For this review, use the dimensioned drawing (mm, ordinates from the lowest corner) and the shaded views. Coordinates: 2 decimals unless noted, no trailing zeros. Loops run counter-clockwise (first coordinate to the right, second up) from the corner with the lowest first, then second, coordinate; pieces in that order, holes last. Notation, with made-up numbers: M 65.5,-7 L 114.5,-7 A28 ccw 114.5,23 Z; hole C 35,-4.5 d10. An arc over 180 degrees is marked long. Write item = value, one per line. Start each with the question number.
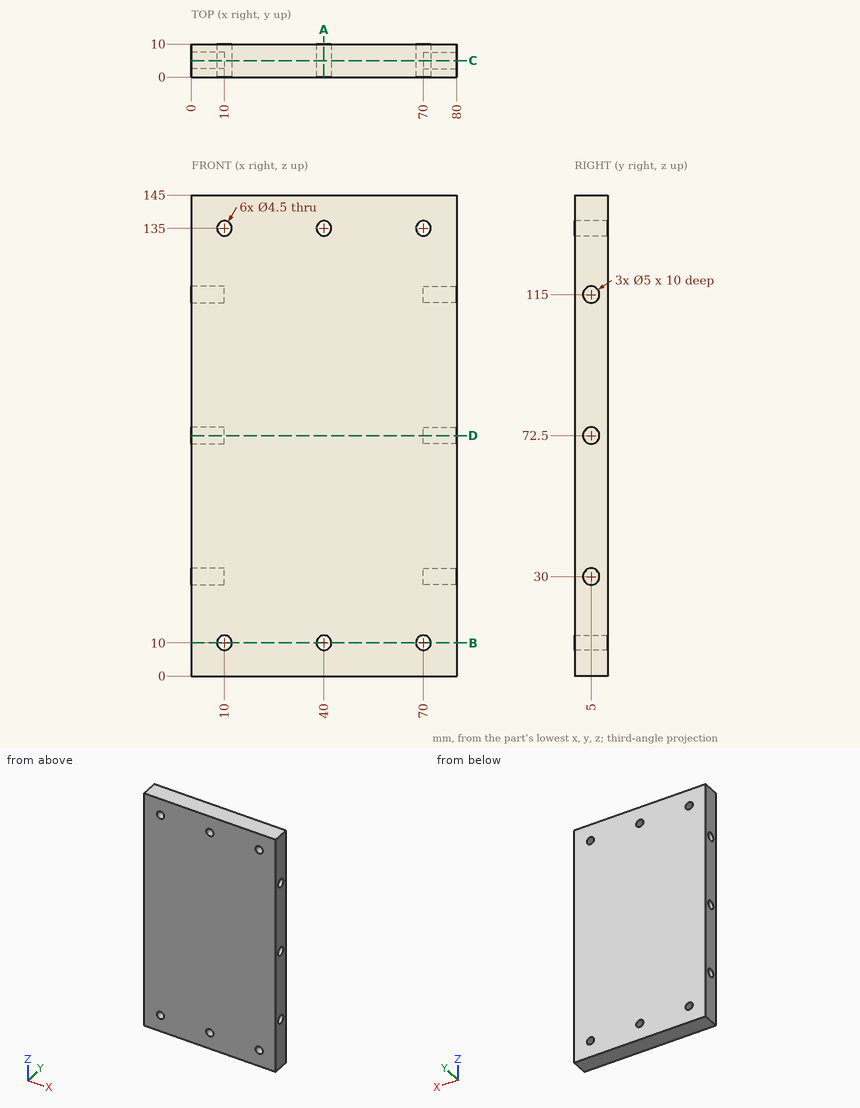
Q1. Add section C-C on y = 5. Give the number of separate pieces and of enclosed holes in the cut face, plus the area to 3 significant figures.
Q2. Clearance check with flat-ended pins moving along their axes: P1, Ø5.5, axis at y = 6, z = 30, coming from the -X side; P2, Ø2.5, axis at x = 10, z = 10, coming from the +Y side; P3, Ø4, axis at y = 5, z = 72.5, coming from the +X side; P4, Ø4, axis at y = 5, z = 115, coming from the -X side. State where each tip first meets the part, or that it passes through.
Q3. Add section A-A on x = 40. State the section outline as (y, z) points.
Q4. To check wall thickness, follow line 1 (X direction, y = 6.75, z = 135); line 2 (Y direction, x = 77, z = 30); line 3 (Z direction, x = 72, y = 1). State the ranges of each line that lie inside material, in increasing order. Write a range as from..to.
Q5. Add section D-D on z = 72.5. State the section outline as (x, y) points.
Q6. Add section B-B on z = 10. State the section outline as (x, y) points.
Values follow:
q1.separate_pieces = 1
q1.enclosed_holes = 6
q1.area = 11,200 mm2
q2.P1 = 0
q2.P2 = through
q2.P3 = 70
q2.P4 = 10
q3.outline = M 0,0 L 10,0 L 10,7.75 L 0,7.75 Z; M 0,12.25 L 10,12.25 L 10,132.75 L 0,132.75 Z; M 0,137.25 L 10,137.25 L 10,145 L 0,145 Z
q4.line_1 = 0..7.75, 12.25..37.75, 42.25..67.75, 72.25..80
q4.line_2 = 0..2.5, 7.5..10
q4.line_3 = 0..8.97, 11.03..133.97, 136.03..145
q5.outline = M 0,0 L 80,0 L 80,2.5 L 70,2.5 L 70,7.5 L 80,7.5 L 80,10 L 0,10 L 0,7.5 L 10,7.5 L 10,2.5 L 0,2.5 Z
q6.outline = M 0,0 L 7.75,0 L 7.75,10 L 0,10 Z; M 12.25,0 L 37.75,0 L 37.75,10 L 12.25,10 Z; M 42.25,0 L 67.75,0 L 67.75,10 L 42.25,10 Z; M 72.25,0 L 80,0 L 80,10 L 72.25,10 Z
